```python
from build123d import *

# Parameters (mm, degrees)
F0_W     = 181.102
F0_H     = 166.878
F1_DEPTH = 75.946
F2_W     = 55.6948
F2_H     = 28.966822
F3_DEPTH = 25.4


with BuildPart() as f1:
    # F0 (on Front) → F1 (new body)
    with BuildSketch(Plane.XZ):
        Rectangle(F0_W, F0_H)
    extrude(amount=F1_DEPTH)

    # F2 (on face) → F3 (cut)
    with BuildSketch(Plane.XY.offset(83.439)):
        with Locations((-62.7036, -61.462589)):
            Rectangle(F2_W, F2_H)
        with Locations((62.7036, -61.462589)):
            Rectangle(F2_W, F2_H)
    extrude(amount=-F3_DEPTH, mode=Mode.SUBTRACT)


solid = f1.part
```
The listing builds one solid part. Answer for the finished solid, in the listing's coordinates (mm). A direction names the side the tool comes from. Coordinates: 2 decimals unless noted, no trailing zeros. Loops run counter-clockwise (first coordinate to the right, second up) from the corner with the lowest first, then second, coordinate; pieces in that order, holes last. Notation, with made-up numbers: M -26.75,-15 L 18.25,-15 A23 ccw 18.25,22 Z; hole C 54.25,3.5 d7. An arc over 180 degrees is marked long. Answer as a JSON object with one key per item and string values. Group by question number.
Item 1: Consider L1, parallel to Y at x = -75.5, z = 75; L2, parallel to X at y = -57.5, z = 61; L3, parallel to Z at x = 81, y = -68. Determine where each line is inside the solid, lowest interval first.
Item 2: Which of the six approach directions +Z, -Z, +X, -X, +Y, -Y give full straight-line access (tool end or side, diameter ignored) to faces 1 (the face through (-90.551, -37, -1)), 2 (the face through (-63, -61, 58.039)), 3 (the face through (62, -61, 58.039))?
Item 3: Each of these flat-tipped pins is pushed along its axis until it touches: P1, Ø7.5, axis at x = 67.5, z = 69, coming from the -Y side; P2, Ø7.5, axis at y = -57, z = 76, coming from the -X side; P3, Ø20.5, axis at y = -64, z = 69.5, coming from the +X side. Where does it stop, or does it pass through?
Item 4: Section A-A (x = -56.5) is taken. Write down the section's boundary in (y, z).
Solved:
{
 "1": {"L1": "y = -46.98 to 0", "L2": "x = -34.86 to 34.86", "L3": "z = -83.44 to 58.04"},
 "2": {"face 1": "+Z, -Z, -X, +Y, -Y", "face 2": "+Z, -X, -Y", "face 3": "+Z, +X, -Y"},
 "3": {"P1": "stops at y = -46.98", "P2": "stops at x = -34.86", "P3": "stops at x = 34.86"},
 "4": {"outline": "M -75.95,-83.44 L 0,-83.44 L 0,83.44 L -46.98,83.44 L -46.98,58.04 L -75.95,58.04 Z"}
}
